from build123d import *

# Parameters (mm, degrees)
F1_DEPTH = 50
F2_DEPTH = 3


with BuildPart() as f1:
    # F0 (on Top) → F1 (new body)
    with BuildSketch(Plane.XY):
        Polygon((-55.9148403892, 33.1440888282), (-56.6610431051, -31.8516278114), (-0.746202716, -64.9957166397), (55.9148403892, -33.1440888282), (56.6610431051, 31.8516278114), (0.746202716, 64.9957166397), align=None)
        Polygon((51.6136988208, -30.5945435338), (-0.688802507, -59.9960461289), (-52.3025013278, -29.4015025952), (-51.6136988208, 30.5945435338), (0.688802507, 59.9960461289), (52.3025013278, 29.4015025952), align=None, mode=Mode.SUBTRACT)
    extrude(amount=F1_DEPTH)

    # F0 (on Top) → F2 (join)
    with BuildSketch(Plane.XY):
        Polygon((-55.9148403892, 33.1440888282), (-56.6610431051, -31.8516278114), (-0.746202716, -64.9957166397), (55.9148403892, -33.1440888282), (56.6610431051, 31.8516278114), (0.746202716, 64.9957166397), align=None)
        Polygon((51.6136988208, -30.5945435338), (-0.688802507, -59.9960461289), (-52.3025013278, -29.4015025952), (-51.6136988208, 30.5945435338), (0.688802507, 59.9960461289), (52.3025013278, 29.4015025952), align=None, mode=Mode.SUBTRACT)
        Polygon((-52.3025013278, -29.4015025952), (-0.688802507, -59.9960461289), (51.6136988208, -30.5945435338), (52.3025013278, 29.4015025952), (0.688802507, 59.9960461289), (-51.6136988208, 30.5945435338), align=None)
    extrude(amount=-F2_DEPTH)


solid = f1.part
Geometry: final body of the model. Coordinates: model frame, mm. A direction names the side the tool comes from. Give positions to 0.01 mm unless a question says otherwise; leave off trailing zeros. Loops run counter-clockwise (first coordinate to the right, second up) from the corner with the lowest first, then second, coordinate; pieces in that order, holes last. Notation, with made-up numbers: M 57.5,88.25 L 80.5,88.25 A34 ccw 80.5,122.25 Z; hole C 76,-1.75 d5. An arc over 180 degrees is marked long. Put each result on its own line as item: value.
1) Reachability of faces 1 (the flat face through (-30, -43, 50)), 2 (the flat face through (-1, 1, 0)) from +Z, -Z, +X, -X, +Y, -Y: full face, straight path, thin tool, end or side. Return the list, or none.
Computed values:
face 1: +Z, +X, -X, +Y, -Y
face 2: +Z
2) Cut plane C-C, the plane y = -4.5. Return the cut outline in (x, z), plus the area to 3 significant figures.
Computed values:
outline: M -56.35,-3 L 56.24,-3 L 56.24,50 L 51.91,50 L 51.91,0 L -52.02,0 L -52.02,50 L -56.35,50 Z
area: 771 mm^2
3) Mould query, pull axis X, two halves, no side actions, for faces 3 (the flat face through (-1, 1, -3)), 4 (the flat face through (-29.1, -48.19, 23.87)), 5 (the flat face through (29.1, 48.19, 23.87)), 6 (the flat face through (-26.134, -44.913, 24.65)). Classes: released by +X, released by -X, zero draft, split by the parting line, or undercut.
Computed values:
face 3: zero draft
face 4: released by -X
face 5: released by +X
face 6: undercut
4) First-contact query: P1, Ø1.5, axis at x = 41.5, z = 21.5, coming from the -Y side; P2, Ø5, axis at y = -29, z = 2.5, coming from the -X side; P3, Ø6, axis at x = -19.5, z = 24, coming from the -Y side; P4, Ø12, axis at x = -38.5, y = -44, coming from the +Z side. Flat tips, straight axial feed; report the tip coordinate or a pass-through.
Computed values:
P1: stops at y = -41.67
P2: stops at x = -56.66
P3: stops at y = -55.66
P4: stops at z = 50
5) Cut plane B-B, the plane x = 34. Return the cut outline in (y, z).
Computed values:
outline: M -45.46,-3 L 45.28,-3 L 45.28,50 L 40.25,50 L 40.25,0 L -40.5,0 L -40.5,50 L -45.46,50 Z
6) Cut plane A-A, the plane z = 35. Return the cut outline in (x, y), plus the area to 3 significant figures.
Computed values:
outline: M -56.66,-31.85 L -0.75,-65 L 55.91,-33.14 L 56.66,31.85 L 0.75,65 L -55.91,33.14 Z; hole M -52.3,-29.4 L -0.69,-60 L 51.61,-30.59 L 52.3,29.4 L 0.69,60 L -51.61,30.59 Z
area: 1,620 mm^2
7) Material intervals for L1, parallel to Z at x = 15, y = 21; L2, parallel to X at y = -6, z = 11; L3, parallel to Y at x = -48, z = 3, sorted ascending. Write a range as from..to.
Computed values:
L1: z = -3..0
L2: x = -56.36..-52.03, 51.9..56.23
L3: y = -36.99..-31.95, 32.63..37.59
